Autodesk Inventor part; units mm, degrees
ref_plane "YZ Plane" through (0, 0, 0) normal (1, 0, 0) x (0, 1, 0)
ref_plane "XZ Plane" through (0, 0, 0) normal (0, 1, 0) x (-1, 0, 0)
ref_plane "XY Plane" through (0, 0, 0) normal (0, 0, 1) x (1, 0, 0)
sketch "Sketch1" plane through (0, 0, 0) normal (0, 0, 1) x (1, 0, 0)
  line L0 (0, 113.8) -> (0, -147.3) construction
  line L1 (-34.4, 0) -> (87.4, 0) construction
  line L2 (-17, 76.5) -> (17, 76.5)
  line L3 (17, 76.5) -> (17, -76.5)
  line L4 (17, -76.5) -> (-17, -76.5)
  line L5 (-17, -76.5) -> (-17, 76.5)
  line L6 (-17, 76.5) -> (17, -76.5) construction
  line L7 (17, 76.5) -> (-17, -76.5) construction
  line L8 (7, 40) -> (17, 40)
  line L9 (17, 40) -> (17, -40)
  line L10 (17, -40) -> (7, -40)
  line L11 (7, -40) -> (7, 40)
  line L12 (7, 40) -> (17, -40) construction
  line L13 (17, 40) -> (7, -40) construction
  line L14 (17, -40) -> (70, -40)
  line L15 (70, -40) -> (70, -110)
  line L16 (70, -110) -> (17, -110)
  line L17 (17, -110) -> (17, -40)
  line L18 (70, -110) -> (20, -110)
  line L19 (20, -110) -> (20, -55)
  line L20 (20, -55) -> (70, -55)
  line L21 (70, -55) -> (70, -110)
  point P0 (0, 0)
  point P1 (12, 0)
  dimension "d4" = 80
  dimension "d5" = 153
  dimension "d6" = 34
  dimension "d7" = 10
  dimension "d10" = 70
  dimension "d11" = 55
  dimension "d12" = 53
  dimension "d13" = 3
extrude "Extrusion3" add sketch "Sketch1" along normal mid plane 50 contours L2 L3 L8 L11 L10 L4 L5
extrude "Extrusion4" add sketch "Sketch1" along normal mid plane 35 contours L3 L14 L15 L20 L19 L16 L17
mirror "Mirror1" about plane through (0, 0, 0) normal (0, 1, 0) of "Extrusion4"
properties part number "17-0028-0085"
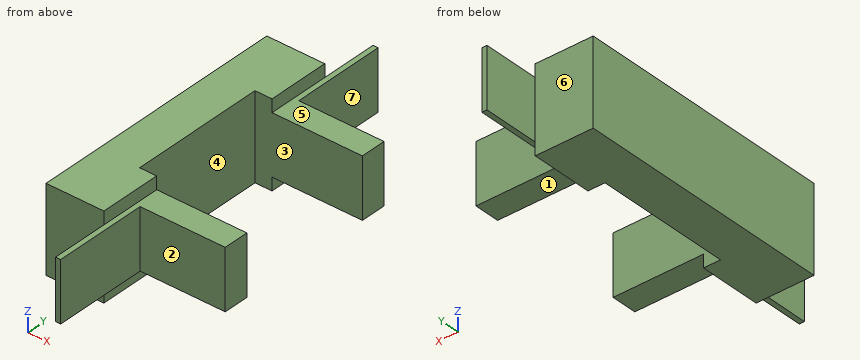
The model under review builds one solid part; all positions refer to its coordinate system, in mm. Face numbers are marked on the shaded views. A direction names the side the tool comes from. Give positions to 0.01 mm unless a question says otherwise; leave off trailing zeros. Write each loop counter-clockwise with the first axis right and the second up, starting at its lowest first coordinate (ties: lowest second). Pieces come first, ordered by that corner, then holes.
(1) The part is to be moulded in two halves that separate along Y. For the marked faces 1, 2 and 3, say which applies: released by +Y, released by -Y, zero draft, split by the parting line, or undercut.
(2) Consider section C-C, the plane y = 9. Give the boundary of the cut face in (x, z).
(3) Consider section A-A, the plane x = 61.5. Give the boundary of the cut face in (y, z), and give its area (3 significant figures).
(4) Consider section B-B, the plane z = -9. Give the boundary of the cut face in (x, y), and give its area (3 significant figures).
(5) For P1, Ø6, axis at y = -60, z = -19.5, coming from the +X side; P2, Ø15, axis at y = -11.5, z = 9.5, coming from the +X side; P3, Ø17, axis at x = 3, z = 5.5, coming from the +Y side; P4, Ø6, axis at x = 15.5, z = 0, coming from the +Y side, all flat-tipped, find the tip position at first contact; note any pin that passes through.
(6) Tool access review of the marked faces 4, 5, 6 and 7: name each direction out of +Z, -Z, +X, -X, +Y, -Y from which nothing blocks a thin tool from reaching the whole face with its end or side.
(7) To check wall thickness, follow L1, parallel to Y at x = 62, z = -1.5; L2, parallel to X at y = 11.5, z = 16; L3, parallel to Y at x = 12.5, z = -13. State the ranges of each line that lie inside material, in increasing order.
(8) Consider section D-D, the plane x = 4. Give the boundary of the cut face in (y, z).
Returned:
1. face 1: zero draft
1. face 2: released by -Y
1. face 3: undercut
2. outline: (-17, -25) - (7, -25) - (7, 25) - (-17, 25) - close
3. outline: (-55, -17.5) - (-40, -17.5) - (-40, 17.5) - (-55, 17.5) - close; (40, -17.5) - (55, -17.5) - (55, 17.5) - (40, 17.5) - close
3. area: 1,050 mm2
4. outline: (-17, -76.5) - (17, -76.5) - (17, -110) - (20, -110) - (20, -55) - (70, -55) - (70, -40) - (7, -40) - (7, 40) - (70, 40) - (70, 55) - (20, 55) - (20, 110) - (17, 110) - (17, 76.5) - (-17, 76.5) - close
4. area: 6,320 mm2
5. P1: stops at x = 20
5. P2: stops at x = 7
5. P3: stops at y = 76.5
5. P4: stops at y = 110
6. face 4: +Z, -Z, +X
6. face 5: +Z, +X, +Y, -Y
6. face 6: +Z, -Z, -X, +Y
6. face 7: +Z, -Z, +X, +Y
7. L1: y = -55 to -40, 40 to 55
7. L2: x = -17 to 7
7. L3: y = -76.5 to -40, 40 to 76.5
8. outline: (-76.5, -25) - (76.5, -25) - (76.5, 25) - (-76.5, 25) - close
